Here's how the part is built. I have some questions about the finished solid (model axes, mm). Face numbers are marked on the shaded views. Round coordinates to 2 decimals unless told otherwise and drop trailing zeros. Order: outer loops, then holes, each group sorted by start corner. A loop starts at its lowest first (then second) coordinate and runs counter-clockwise, first axis right, second up.
```python
from build123d import *

# Parameters (mm, degrees)
F0_R     = 28
F0_R_2   = 26
F1_DEPTH = 4
F2_R     = 29
F2_R_2   = 28
F3_DEPTH = 15
F4_R     = 0.5


with BuildPart() as f1:
    # F0 (on Top) → F1 (new body)
    with BuildSketch(Plane.XY):
        Circle(F0_R)
        Circle(F0_R_2, mode=Mode.SUBTRACT)
    extrude(amount=F1_DEPTH)

    # F2 (on face) → F3 (join)
    with BuildSketch(Plane.XY.offset(4)):
        Circle(F2_R)
        Circle(F2_R_2, mode=Mode.SUBTRACT)
    extrude(amount=-F3_DEPTH)

    # F4
    f4_edges = [f1.edges().sort_by_distance(p)[0] for p in [
        (-26, 0, 4),
        (-29, 0, 4),
    ]]
    fillet(f4_edges, radius=F4_R)


solid = f1.part
```
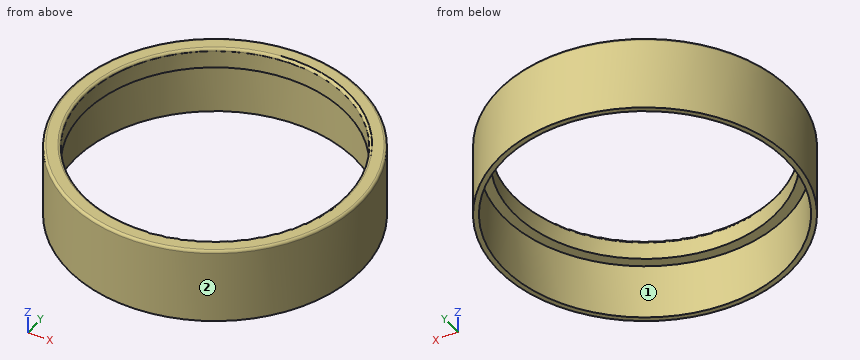
1) I need wall thicknesses on line 1 (Y direction, x = 0, z = -3); line 2 (Y direction, x = 0, z = 2.1); line 3 (Z direction, x = 14, y = -23). Which ranges of each line are inside material? Lowest first, please.
2) We'd pull the mould along X, two halves only. Please class the marked faces 1 and 2: +X half, -X half, draft (parallel to the pull), parting line (faces both ways), or undercut.
3) If we section it at D-D (z = -9.25): Write out the boundary of the cut face in (x, y).
4) I'm going to push flat-ended pins straight in: pin 1 (2 mm diameter, centred on y = -15, z = 0, fed in from -X); pin 2 (6 mm diameter, centred on x = 10.5, z = -4.5, fed in from +Y); pin 3 (3 mm diameter, centred on y = -13, z = -6, fed in from -X). Where does each tip first touch, or does it pass through?
5) If we section it at A-A (y = 0): Write out the boundary of the cut face in (x, z).
6) If we section it at C-C (z = 1.75): Write out the boundary of the cut face in (x, y).
Solutions:
1. line 1: y = -29 to -28, 28 to 29
1. line 2: y = -29 to -26, 26 to 29
1. line 3: z = 0 to 4
2. face 1: undercut
2. face 2: parting line
3. outline: circle Ø58 at (0, 0); hole circle Ø56 at (0, 0)
4. pin 1: stops at x = -25.4
4. pin 2: stops at y = 28.01
4. pin 3: stops at x = -26.62
5. outline: (-29, -11) - (-28, -11) - (-28, 0) - (-26, 0) - (-26, 3.5) arc R0.5 ccw to (-26.5, 4) - (-28.5, 4) arc R0.5 ccw to (-29, 3.5) - close; (26, 0) - (28, 0) - (28, -11) - (29, -11) - (29, 3.5) arc R0.5 ccw to (28.5, 4) - (26.5, 4) arc R0.5 ccw to (26, 3.5) - close
6. outline: circle Ø58 at (0, 0); hole circle Ø52 at (0, 0)
